```python
from build123d import *

# Parameters (mm, degrees)
F1_W      = 50
F1_H      = 50
F2_DEPTH  = 25
F3_ANGLE  = 45
F0_W      = 100
F0_H      = 100
F2_FACE_W = 50
F2_FACE_H = 50
F4_DEPTH  = 25


with BuildPart() as f2:
    # F1 (on Front) → F2 (new body)
    with BuildSketch(Plane.XZ):
        Rectangle(F1_W, F1_H)
    extrude(amount=F2_DEPTH)


with BuildPart() as f2_1:
    # F3: moved
    add(f2.part.rotate(Axis((-25, -25, 0), (0, 0, -1)), F3_ANGLE))

    # F0 (on Front) + F2_face (on face) → F4 (join)
    with BuildSketch(Plane.XZ):
        Rectangle(F0_W, F0_H)
    with BuildSketch(Plane(origin=(-7.3223304703, -42.6776695297, 0), x_dir=(0.7071067812, -0.7071067812, 0), z_dir=(-0.7071067812, -0.7071067812, 0))):
        Rectangle(F2_FACE_W, F2_FACE_H)
    extrude(amount=F4_DEPTH, dir=(0, -1, 0))


solid = f2_1.part
```
Part model, mm, in its own coordinate system. A direction names the side the tool comes from. Round coordinates to 2 decimals unless told otherwise and drop trailing zeros. Write each loop counter-clockwise with the first axis right and the second up, starting at its lowest first coordinate (ties: lowest second). Pieces come first, ordered by that corner, then holes. Notation, with made-up numbers: M 64.5,-14.5 L 116.5,-14.5 A7 cw 116.5,-5.5 Z; hole C 80.25,80.25 d11. An arc over 180 degrees is marked long. Answer as CSV lines item,"result". Start each with the question number.
1) Which spindle directions (+Z, -Z, +X, -X, +Y, -Y) get a long thin tool onto all of the face, cutting with end or side? Do faces 4 (the face through (-25, -37, 0)), 5 (the face through (1, -46, -25)), 6 (the face through (10.355, -73, 0)), 7 (the face through (1, -46, 25)). Say none if no direction does.
2) Drop flat-ended pins along their axis: pin 1 (8 mm diameter, centred on x = -6, z = -31.5, fed in from -Y); pin 2 (16 mm diameter, centred on x = 11, y = -67.5, fed in from +Z); pin 3 (20 mm diameter, centred on y = -68.5, z = 3.5, fed in from +X). Give the stop position or say it passes through.
3) Band-saw the part on A-A (x = -13). List the corners of the cut face in (y, z), then the cut area to 3 significant figures.
4) Band-saw the part on B-B (x = 15). List the corners of the cut face in (y, z), then the cut area to 3 significant figures.
5) Band-saw the part on D-D (y = -78.5). List the corners of the cut face in (x, z), then the cut area to 3 significant figures.
6) Band-saw the part on C-C (z = -7). List the corners of the cut face in (x, y), then the cut area to 3 significant figures.
7) Drill centre lines: L1, parallel to Z at x = -13.5, y = -38; L2, parallel to Y at x = -26.5, z = -8.5; L3, parallel to X at y = -74, z = -19. Where is each one in solid material? Low to high.
8) Mould opens along Y. For faces 1 (the face through (19.07, -33.715, 0.35)), 2 (the face through (-1, -12, 50)), 3 (the face through (-8, -67, 0)) say: +Y half, -Y half, draft (parallel to the pull), parting line (faces both ways), or undercut.
Worked out:
1,face 4,"+Z, -Z, -X, -Y"
1,face 5,"-Z, +X, -X, -Y"
1,face 6,"+Z, -Z, +X, -Y"
1,face 7,"+Z, +X, -X, -Y"
2,pin 1,"y = -25"
2,pin 2,"z = 25"
2,pin 3,"x = 12.21"
3,outline,"M -62,-25 L -25,-25 L -25,-50 L 0,-50 L 0,50 L -25,50 L -25,25 L -62,25 Z"
3,area,"4,350 mm²"
4,outline,"M -55.71,-25 L -29.64,-25 L -29.64,25 L -55.71,25 Z; M -25,-50 L 0,-50 L 0,50 L -25,50 Z"
4,area,"3,800 mm²"
5,outline,"M 3.5,-25 L 10.36,-25 L 10.36,25 L 3.5,25 Z"
5,area,"343 mm²"
6,outline,"M -50,-25 L -25,-25 L -25,-50 L 10.36,-85.36 L 10.36,-60.36 L 28.03,-42.68 L 10.36,-25 L 50,-25 L 50,0 L -50,0 Z"
6,area,"4,320 mm²"
7,L1,"-25 to 25"
7,L2,"-25 to 0"
7,L3,"-1 to 10.36"
8,face 1,"undercut"
8,face 2,"draft"
8,face 3,"-Y half"
